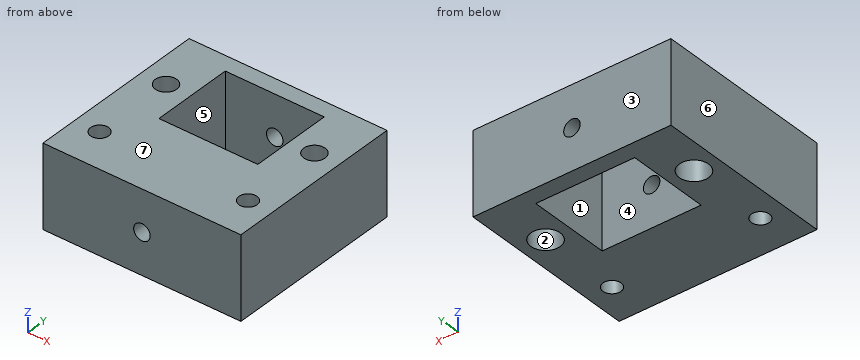
```python
from build123d import *

# Parameters (mm, degrees)
SKETCH2_W           = 60
SKETCH2_H           = 25
BOSS_EXTRUDE1_DEPTH = 55
CUT_EXTRUDE1_REACH  = 27
SKETCH3_W           = 30
SKETCH3_H           = 25
SKETCH4_R           = 2.5
CUT_EXTRUDE2_DEPTH  = 56
SKETCH5_R           = 3.25
SKETCH5_R_2         = 2.75
CUT_EXTRUDE3_DEPTH  = 26
SKETCH9_R           = 4.45
CUT_EXTRUDE7_DEPTH  = 11.5


with BuildPart() as part:
    # Sketch2 → Boss-Extrude1 (new body)
    with BuildSketch(Plane(origin=(0, 0, 0), x_dir=(1, 0, 0), z_dir=(0, 1, 0))):
        with Locations((30, 12.5)):
            Rectangle(SKETCH2_W, SKETCH2_H)
    extrude(amount=BOSS_EXTRUDE1_DEPTH)

    # Sketch3 → Cut-Extrude1 (cut, up to next)
    with BuildSketch(Plane.XY, mode=Mode.PRIVATE) as cut_extrude1_sk1:
        with Locations((30, 37.5)):
            Rectangle(SKETCH3_W, SKETCH3_H)
    cut_extrude1_tool1 = extrude(cut_extrude1_sk1.sketch, amount=-CUT_EXTRUDE1_REACH, mode=Mode.PRIVATE) & part.part
    add(cut_extrude1_tool1.solids().sort_by_distance((30, 37.5, 0))[0], mode=Mode.SUBTRACT)

    # Sketch4 → Cut-Extrude2 (cut, through all)
    with BuildSketch(Plane(origin=(0, 55, 0), x_dir=(1, 0, 0), z_dir=(0, 1, 0))):
        with Locations((30, 12.5)):
            Circle(SKETCH4_R)
    extrude(amount=-CUT_EXTRUDE2_DEPTH, mode=Mode.SUBTRACT)

    # Sketch5 → Cut-Extrude3 (cut, through all)
    with BuildSketch(Plane.XY):
        with Locations((7.5, 37)):
            Circle(SKETCH5_R)
        with Locations((7.5, 12)):
            Circle(SKETCH5_R_2)
        with Locations((52.5, 12)):
            Circle(SKETCH5_R_2)
        with Locations((52.5, 37)):
            Circle(SKETCH5_R)
    extrude(amount=-CUT_EXTRUDE3_DEPTH, mode=Mode.SUBTRACT)

    # Sketch9 → Cut-Extrude7 (cut)
    with BuildSketch(Plane(origin=(0, 0, -25), x_dir=(-1, 0, 0), z_dir=(0, 0, -1))):
        with Locations((-52.5, 37)):
            Circle(SKETCH9_R)
        with Locations((-7.5, 37)):
            Circle(SKETCH9_R)
    extrude(amount=-CUT_EXTRUDE7_DEPTH, mode=Mode.SUBTRACT)


solid = part.part
```
Here's how the part is built. I have some questions about the finished solid (model axes, mm). Face numbers are marked on the shaded views. A direction names the side the tool comes from. Coordinates: 2 decimals unless noted, no trailing zeros. Order: outer loops, then holes, each group sorted by start corner. A loop starts at its lowest first (then second) coordinate and runs counter-clockwise, first axis right, second up.
1) Imagine slicing it at C-C on y = 29. List the corners of the cut face in (x, z) for me.
2) Imagine slicing it at A-A on z = -12.5. List the corners of the cut face in (x, y) for me, and give its area (3 significant figures).
3) Imagine slicing it at D-D on z = -21. List the corners of the cut face in (x, y) for me.
4) We'd pull the mould along X, two halves only. Please class the marked faces 4, 5, 6 and 7: +X half, -X half, draft (parallel to the pull), parting line (faces both ways), or undercut.
5) Which directions (+Z, -Z, +X, -X, +Y, -Y) give clear straight access to the entire face, cutting with the end or side of a thin tool? Please do the marked faces 1, 2 and 3.
6) I need wall thicknesses on line 1 (Y direction, x = 7.5, z = -21.25); line 2 (Z direction, x = 30, y = 12.5); line 3 (Y direction, x = 20, z = -0.75). Which ranges of each line are inside material? Lowest first, please.
7) Will these pins go through, and if not, where does the flat tip stop? pin 1 (3 mm diameter, centred on x = 27.5, y = 13, fed in from +Z); pin 2 (8 mm diameter, centred on x = 52.5, y = 37, fed in from -Z).
8) Imagine slicing it at B-B on y = 12. List the corners of the cut face in (x, z) for me.
Response values:
1. outline: (0, -25) - (15, -25) - (15, 0) - (0, 0) - close; (45, -25) - (60, -25) - (60, 0) - (45, 0) - close
2. outline: (0, 0) - (27.5, 0) - (27.5, 25) - (15, 25) - (15, 50) - (27.5, 50) - (27.5, 55) - (0, 55) - close; (32.5, 0) - (60, 0) - (60, 55) - (32.5, 55) - (32.5, 50) - (45, 50) - (45, 25) - (32.5, 25) - close; hole circle Ø6.5 at (7.5, 37); hole circle Ø5.5 at (7.5, 12); hole circle Ø6.5 at (52.5, 37); hole circle Ø5.5 at (52.5, 12)
2. area: 2,290 mm2
3. outline: (0, 0) - (60, 0) - (60, 55) - (0, 55) - close; hole circle Ø8.9 at (7.5, 37); hole circle Ø5.5 at (7.5, 12); hole (15, 25) - (45, 25) - (45, 50) - (15, 50) - close; hole circle Ø8.9 at (52.5, 37); hole circle Ø5.5 at (52.5, 12)
4. face 4: undercut
4. face 5: undercut
4. face 6: -X half
4. face 7: draft
5. face 1: +Z, -Z
5. face 2: -Z
5. face 3: +Z, -Z, +X, -X, +Y
6. line 1: y = 0 to 9.25, 14.75 to 32.55, 41.45 to 55
6. line 2: z = -25 to -15, -10 to 0
6. line 3: y = 0 to 25, 50 to 55
7. pin 1: stops at z = 0
7. pin 2: stops at z = -13.5
8. outline: (0, -25) - (4.75, -25) - (4.75, 0) - (0, 0) - close; (10.25, -25) - (49.75, -25) - (49.75, 0) - (10.25, 0) - close; (55.25, -25) - (60, -25) - (60, 0) - (55.25, 0) - close; hole circle Ø5 at (30, -12.5)
